Could you check a few things on this drawing? It's one solid part, dimensions in mm from its lowest x, y, z. Give positions to 0.01 mm unless a question says otherwise; leave off trailing zeros. Loops run counter-clockwise (first coordinate to the right, second up) from the corner with the lowest first, then second, coordinate; pieces in that order, holes last. Notation, with made-up numbers: (-0.5, 38) - (26.5, 38) arc R22 cw to (26.5, 51) - close; hole circle Ø6 at (88.5, -8). An arc over 180 degrees is marked (long way). Write item = value, one per line.
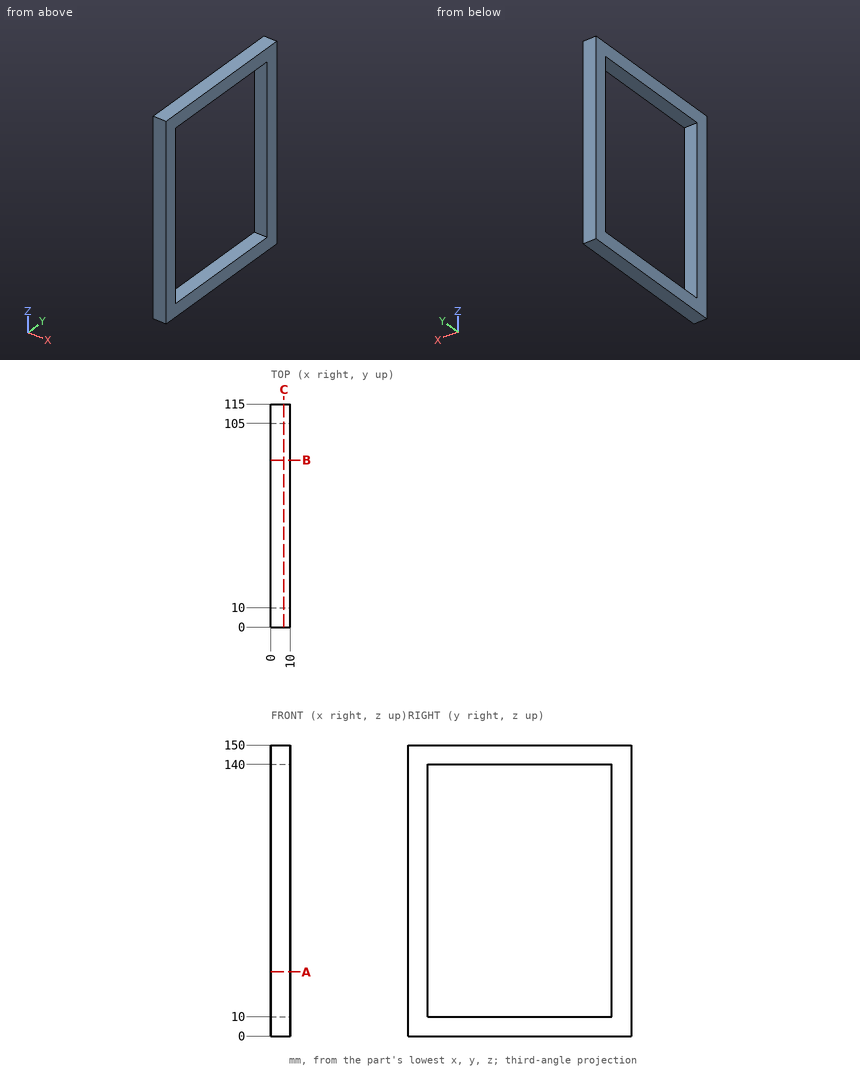
Q1. Imagine slicing it at A-A, the plane z = 33. Write out the boundary of the cut face in (x, y).
Output:
outline = (0, 0) - (10, 0) - (10, 10) - (0, 10) - close; (0, 105) - (10, 105) - (10, 115) - (0, 115) - close
Q2. Imagine slicing it at B-B, the plane y = 86. Write out the boundary of the cut face in (x, z), then the cut area to 3 significant figures.
Output:
outline = (0, 0) - (10, 0) - (10, 10) - (0, 10) - close; (0, 140) - (10, 140) - (10, 150) - (0, 150) - close
area = 200 mm2
Q3. I need wall thicknesses on L1, parallel to Y at x = 4, z = 139.5; L2, parallel to Z at x = 1, y = 41. Which ranges of each line are inside material? Lowest first, please.
Output:
L1 = 0 to 10, 105 to 115
L2 = 0 to 10, 140 to 150
Q4. Imagine slicing it at C-C, the plane x = 6.75. Write out the boundary of the cut face in (y, z).
Output:
outline = (0, 0) - (115, 0) - (115, 150) - (0, 150) - close; hole (10, 10) - (105, 10) - (105, 140) - (10, 140) - close
